Design review of the part built by this model. Coordinates are the model's own, in mm. A direction names the side the tool comes from. Coordinates: 2 decimals unless noted, no trailing zeros. Write each loop counter-clockwise with the first axis right and the second up, starting at its lowest first coordinate (ties: lowest second). Pieces come first, ordered by that corner, then holes. Notation, with made-up numbers: M -25,17 L -6,17 A15 ccw -6,21 Z; hole C 53,28 d8. An arc over 180 degrees is marked long. One line per question, with ' | ' between items.
from build123d import *

# Parameters (mm, degrees)
SKETCH026_W     = 95
SKETCH026_H     = 95
PAD018_DEPTH    = 5
PAD019_DEPTH    = 95
SKETCH028_R     = 30
POCKET008_DEPTH = 95.001
FILLET020_R     = 5
FILLET021_R     = 2


with BuildPart() as part:
    # Sketch026 → Pad018 (new body)
    with BuildSketch(Plane.XY):
        Rectangle(SKETCH026_W, SKETCH026_H)
    extrude(amount=PAD018_DEPTH)

    # Sketch027 (on DatumPlane) → Pad019 (join)
    with BuildSketch(Plane(origin=(0, 47.5, 0), x_dir=(-1, 0, 0), z_dir=(0, 1, 0))):
        Polygon((-47, 5), (-17, 56.961524), (-14, 56.961524), (-44, 5), align=None)
        Polygon((-39, 5), (-9, 56.961524), (-6, 56.961524), (-36, 5), align=None)
        Polygon((-26, 5), (4, 56.961524), (7, 56.961524), (-23, 5), align=None)
        Polygon((-8, 5), (22, 56.961524), (25, 56.961524), (-5, 5), align=None)
        Polygon((10, 5), (40, 56.961524), (43, 56.961524), (13, 5), align=None)
    extrude(amount=-PAD019_DEPTH)

    # Sketch028 (on DatumPlane) → Pocket008 (cut, through all)
    with BuildSketch(Plane.YZ.offset(47.5)):
        with Locations((0, 60)):
            Circle(SKETCH028_R)
    extrude(amount=-POCKET008_DEPTH, mode=Mode.SUBTRACT)

    # Fillet020
    fillet020_edges = [part.edges().sort_by_distance(p)[0] for p in [
        (15.5, -47.5, 56.961524),
        (15.5, -29.845731, 56.961524),
        (7.5, -47.5, 56.961524),
        (7.5, -29.845731, 56.961524),
        (-5.5, -47.5, 56.961524),
        (-5.5, -29.845731, 56.961524),
        (-23.5, -47.5, 56.961524),
        (-23.5, -29.845731, 56.961524),
        (-41.5, -47.5, 56.961524),
        (-41.5, -29.845731, 56.961524),
        (15.5, 29.845731, 56.961524),
        (15.5, 47.5, 56.961524),
        (7.5, 29.845731, 56.961524),
        (7.5, 47.5, 56.961524),
        (-5.5, 29.845731, 56.961524),
        (-5.5, 47.5, 56.961524),
        (-23.5, 29.845731, 56.961524),
        (-23.5, 47.5, 56.961524),
        (-41.5, 29.845731, 56.961524),
        (-41.5, 47.5, 56.961524),
    ]]
    fillet(fillet020_edges, radius=FILLET020_R)

    # Fillet021
    fillet021_edges = [part.edges().sort_by_distance(p)[0] for p in [
        (0, 47.5, 0),
        (47.5, 0, 0),
        (0, -47.5, 0),
        (-47.5, 0, 0),
    ]]
    fillet(fillet021_edges, radius=FILLET021_R)


with BuildPart() as part_1:
    # Body012 placement: moved
    add(part.part.moved(Location((-47, 233, 0))))


solid = part_1.part
1. Draft analysis for pull direction Y (two halves, no side actions). For faces 4 (the face through (-51.93, 202, 55.91)), 5 (the face through (-52, 195, 56.962)), 6 (the face through (-69.75, 186.93, 55.46)), 7 (the face through (-51.75, 279.07, 55.46)), state which applies: pulls with the +Y half, pulls with the -Y half, needs draft (parallel to the pull), parting line crosses it, or undercut.
Answer sheet:
face 4: undercut | face 5: needs draft | face 6: pulls with the -Y half | face 7: pulls with the +Y half
2. Tool access review of faces 1 (the face through (-88, 271, 56.962)), 2 (the face through (-69.93, 264, 55.91)), 3 (the face through (-68.457, 233.665, 24.844)): name each direction out of +Z, -Z, +X, -X, +Y, -Y from which nothing blocks a thin tool from reaching the whole face with its end or side.
Answer sheet:
face 1: +Z, +X, -X, +Y, -Y | face 2: +Z, +X, -X | face 3: +Y, -Y
3. To check wall thickness, follow line 1 along X through (y, z) = (203, 12); line 2 along Z through (x, y) = (-37, 190); line 3 along Z through (x, y) = (-21.5, 254). State the ranges of each line that lie inside material, in increasing order. Write a range as [from, to].
Answer sheet:
line 1: [-64.04, -61.04], [-46.04, -43.04], [-28.04, -25.04], [-15.04, -12.04], [-7.04, -4.04] | line 2: [0, 5], [27.52, 32.71], [50.03, 55.23] | line 3: [0, 5.87], [23.19, 28.38], [37.04, 38.58]
4. Take a section at B-B (x = -63). Write out the cut boundary in (y, z).
Answer sheet:
outline: M 185.5,2 A2 ccw 187.5,0 L 278.5,0 A2 ccw 280.5,2 L 280.5,5 L 185.5,5 Z; M 185.5,10.2 L 280.5,10.2 L 280.5,15.39 L 185.5,15.39 Z; M 185.5,41.37 L 209.48,41.37 A30 cw 206.17,46.57 L 185.5,46.57 Z; M 256.52,41.37 L 280.5,41.37 L 280.5,46.57 L 259.83,46.57 A30 cw Z
5. Take a section at C-C (x = -77). Write out the cut boundary in (y, z).
Answer sheet:
outline: M 185.5,2 A2 ccw 187.5,0 L 278.5,0 A2 ccw 280.5,2 L 280.5,5 L 185.5,5 Z; M 185.5,34.44 L 217.29,34.44 A30 cw 210.97,39.64 L 185.5,39.64 Z; M 248.71,34.44 L 280.5,34.44 L 280.5,39.64 L 255.03,39.64 A30 cw Z
6. Take a section at D-D (z = 8.5). Write out the cut boundary in (x, y).
Answer sheet:
outline: M -62.02,185.5 L -59.02,185.5 L -59.02,280.5 L -62.02,280.5 Z; M -44.02,185.5 L -41.02,185.5 L -41.02,280.5 L -44.02,280.5 Z; M -26.02,185.5 L -23.02,185.5 L -23.02,280.5 L -26.02,280.5 Z; M -13.02,185.5 L -10.02,185.5 L -10.02,280.5 L -13.02,280.5 Z; M -5.02,185.5 L -2.02,185.5 L -2.02,280.5 L -5.02,280.5 Z
7. Insertion check: pin 1 Ø8 at (x, y) = (-73.5, 216.5) entering from +Z; pin 2 Ø4 at (x, y) = (-6, 221.5) entering from +Z; pin 3 Ø4.5 at (x, y) = (-49.5, 245.5) entering from +Z. Each pin has a flat end and moves straight along its axis. Give the tip position at first contact, or say it passes through.
Answer sheet:
pin 1: z = 37.47 | pin 2: z = 18.86 | pin 3: z = 27.08
8. Take a section at A-A (x = -6). Write out the cut boundary in (y, z), then the cut area to 3 significant figures.
Answer sheet:
outline: M 185.5,2 A2 ccw 187.5,0 L 278.5,0 A2 ccw 280.5,2 L 280.5,5 L 185.5,5 Z; M 185.5,10.2 L 280.5,10.2 L 280.5,15.39 L 185.5,15.39 Z | area: 967 mm^2
